Read the model definition and answer for the solid it produces. Units are mm, in the model's axes. A direction names the side the tool comes from. Coordinates: 2 decimals unless noted, no trailing zeros. Write each loop counter-clockwise with the first axis right and the second up, starting at its lowest first coordinate (ties: lowest second). Pieces come first, ordered by that corner, then holes. Notation, with made-up numbers: (39.5, 13.25) -> (91.5, 13.25) arc R22 ccw to (91.5, 51.25) -> close; hole circle Ø8 at (22, -10.5). An arc over 180 degrees is marked (long way). Return JSON: item names as keys, results as strings.
from build123d import *

# Parameters (mm, degrees)
F2_R     = 4.7625
F3_DEPTH = 9.525
F4_R     = 1.5875
F5_DEPTH = 21.844


with BuildPart() as f1:
    # F0 (on Front) → F1 (revolve)
    with BuildSketch(Plane.XZ):
        Polygon((0, 62.927276), (0, 0), (30.991441, 6.508361), (30.991441, 25.977967), (8.01147, 25.977967), (8.01147, 62.927276), align=None)
    revolve(axis=Axis((0, 0, 31.463638), (0, 0, -1)))

    # F2 (on face) → F3 (cut)
    with BuildSketch(Plane.XY.offset(62.927276)):
        Circle(F2_R)
    extrude(amount=-F3_DEPTH, mode=Mode.SUBTRACT)

    # F4 (on Top) → F5 (cut)
    with BuildSketch(Plane.XY):
        Circle(F4_R)
    extrude(amount=F5_DEPTH, mode=Mode.SUBTRACT)


solid = f1.part
1. The part is cut by section C-C (z = 20). Determine the outline of the cut face in (x, y) (1 decimal).
Taken from the geometry:
{"outline": "circle Ø62 at (0, 0); hole circle Ø3.2 at (0, 0)"}
2. The part is cut by section A-A (x = 0). Determine the outline of the cut face in (y, z).
Taken from the geometry:
{"outline": "(-30.99, 6.51) -> (-1.59, 0.33) -> (-1.59, 21.84) -> (1.59, 21.84) -> (1.59, 0.33) -> (30.99, 6.51) -> (30.99, 25.98) -> (8.01, 25.98) -> (8.01, 62.93) -> (4.76, 62.93) -> (4.76, 53.4) -> (-4.76, 53.4) -> (-4.76, 62.93) -> (-8.01, 62.93) -> (-8.01, 25.98) -> (-30.99, 25.98) -> close"}
3. Flat-ended cylindrical pins translate along their axes: pin 1 Ø12 at (y, z) = (8.5, 22.5) entering from +X; pin 2 Ø1.6 at (x, y) = (0, -0.5) entering from -Z; pin 3 Ø8 at (x, z) = (6, 26) entering from -Y. Find the tip coordinate at first contact, or state that the pin passes through.
Taken from the geometry:
{"pin 1": "stops at x = 30.89", "pin 2": "stops at z = 21.84", "pin 3": "stops at y = -30.93"}
4. For a pull along Y with two mould halves and no side action, classify faces 3 (the face through (-3.78, -2.9, 58.23)), 4 (the face through (29.56, -9.31, 16.38)), 5 (the face through (5, 0, 62.927)), 6 (the face through (-0.34, -1.55, 10.94)) as +Y half, -Y half, draft (parallel to the pull), parting line (faces both ways), or undercut.
Taken from the geometry:
{"face 3": "undercut", "face 4": "parting line", "face 5": "draft", "face 6": "undercut"}
5. Consider L1, parallel to Y at x = 0, z = 58; L2, parallel to Y at x = 0, z = 13. Determine where each line is inside the solid, lowest interval first.
Taken from the geometry:
{"L1": "y = -8.01 to -4.76, 4.76 to 8.01", "L2": "y = -30.99 to -1.59, 1.59 to 30.99"}
6. A tool of negligible diameter and unlimited length cuts with its end or side. For faces 1 (the face through (0, 0, 21.844)), 2 (the face through (0, 0, 53.402)), from which of +Z, -Z, +X, -X, +Y, -Y can it reach the whole face along a straight path? Write none if from no direction.
Taken from the geometry:
{"face 1": "-Z", "face 2": "+Z"}
